```python
from build123d import *

# Parameters (mm, degrees)
SKETCH001_W = 6.3
SKETCH001_H = 1.5


with BuildPart() as y_belt_seg2:
    # Sweep001: sweep along a path in Sketch002
    with BuildLine(Plane.YZ) as sweep001_path:
        Line((-16.5, 34.3), (-2, 34.3))
        ThreePointArc((-2, 34.3), (-1.787868, 34.212132), (-1.7, 34))
        Line((-1.7, 34), (-1.7, 25.1))
        ThreePointArc((-1.7, 25.1), (-1.787868, 24.887868), (-2, 24.8))
        Line((-2, 24.8), (-16.5, 24.8))
        ThreePointArc((-16.5, 24.8), (-16.821394, 24.916978), (-16.992404, 25.213176))
        Line((-16.992404, 25.213176), (-18.285606, 32.547297))
        ThreePointArc((-18.285606, 32.547297), (-18.969647, 33.732089), (-20.255221, 34.2))
        Line((-20.255221, 34.2), (-32.255221, 34.2))
    # Sketch001 → Sweep001 (sweep)
    with BuildSketch(Plane(origin=(0, -16.5, 35.05), x_dir=(1, 0, 0), z_dir=(0, -1, 0))):
        Rectangle(SKETCH001_W, SKETCH001_H)
    sweep(path=sweep001_path.line)


with BuildPart() as part_mirroring:
    # Part__Mirroring: instance of y-belt-seg2
    add(y_belt_seg2.part.mirror(Plane(origin=(0, 0, 0), x_dir=(1, 0, 0), z_dir=(0, 1, 0))))


with BuildPart() as y_belt:
    # Sweep: sweep along a path in Sketch
    with BuildLine(Plane.YZ) as sweep_path:
        Line((16.5, 34.3), (131.990476, 34.499992))
        ThreePointArc((131.990476, 34.499992), (137.49996, 29.021053), (132.032583, 23.500097))
        Line((132.032583, 23.500097), (-138.041883, 21.900109))
        ThreePointArc((-138.041883, 21.900109), (-144.278585, 28.081635), (-138.078613, 34.3))
        Line((-138.078613, 34.3), (-16.5, 34.3))
    # Sketch001 → Sweep (sweep)
    with BuildSketch(Plane(origin=(0, -16.5, 35.05), x_dir=(1, 0, 0), z_dir=(0, -1, 0))):
        Rectangle(SKETCH001_W, SKETCH001_H)
    sweep(path=sweep_path.line)

    # Fusion: union Part__Mirroring, y-belt-seg2
    add(part_mirroring.part)
    add(y_belt_seg2.part)


solid = y_belt.part
```
Source: CAD feature listing. Evaluate the final solid. Frame: model axes, mm. A direction names the side the tool comes from. Round coordinates to 2 decimals unless told otherwise and drop trailing zeros. Write each loop counter-clockwise with the first axis right and the second up, starting at its lowest first coordinate (ties: lowest second). Pieces come first, ordered by that corner, then holes. Notation, with made-up numbers: M 32.25,-29 L 57.25,-29 A14 ccw 57.25,-21 Z; hole C 33,72.5 d10. An arc over 180 degrees is marked long. Answer as a JSON object with one key per item and string values. Group by question number.
(1) Section query B-B on y = -66.5. Output: boundary loops of the cut face in (x, z), then the cut area to 3 significant figures.
(2) Section query A-A on z = 28.1. Output: boundary loops of the cut face in (x, y).
(3) First-contact query: pin 1 (1.9 mm diameter, centred on x = 1.5, z = 31.5, fed in from +Y); pin 2 (1.9 mm diameter, centred on x = -0.5, y = 10, fed in from -Z); pin 3 (1.5 mm diameter, centred on x = 2, y = 66, fed in from +Z). Flat tips, straight axial feed; report the tip coordinate or a pass-through.
(4) Section query C-C on y = -10. Output: boundary loops of the cut face in (x, z), then the cut area to 3 significant figures.
(5) Reachability of faces 1 (the flat face through (0, -0.2, 29)), 2 (the flat face through (0, 9, 34.3)) from +Z, -Z, +X, -X, +Y, -Y: full face, straight path, thin tool, end or side. Return the list, or none.
(6) Ray query, line 1 (Z direction, x = 2, y = -132); line 2 (Z direction, x = -2.5, y = 8); line 3 (Y direction, x = 2, z = 31.5). Return the intervals inside material, ascending. Write a range as [from, to].
Computed values:
{
 "1": {"outline": "M -3.15,20.82 L 3.15,20.82 L 3.15,22.32 L -3.15,22.32 Z; M -3.15,34.3 L 3.15,34.3 L 3.15,35.8 L -3.15,35.8 Z", "area": "18.9 mm^2"},
 "2": {"outline": "M -3.15,-145.78 L 3.15,-145.78 L 3.15,-144.28 L -3.15,-144.28 Z; M -3.15,-19.02 L 3.15,-19.02 L 3.15,-17.5 L -3.15,-17.5 Z; M -3.15,-1.7 L 3.15,-1.7 L 3.15,-0.2 L -3.15,-0.2 Z; M -3.15,0.2 L 3.15,0.2 L 3.15,1.7 L -3.15,1.7 Z; M -3.15,17.5 L 3.15,17.5 L 3.15,19.02 L -3.15,19.02 Z; M -3.15,137.43 L 3.15,137.43 L 3.15,138.94 L -3.15,138.94 Z"},
 "3": {"pin 1": "y = 138.83", "pin 2": "z = 21.27", "pin 3": "z = 35.89"},
 "4": {"outline": "M -3.15,21.16 L 3.15,21.16 L 3.15,22.66 L -3.15,22.66 Z; M -3.15,23.3 L 3.15,23.3 L 3.15,24.8 L -3.15,24.8 Z; M -3.15,34.3 L 3.15,34.3 L 3.15,35.8 L -3.15,35.8 Z", "area": "28.4 mm^2"},
 "5": {"face 1": "+Z, +X, -X", "face 2": "+X, -X"},
 "6": {"line 1": "[20.44, 21.94], [34.3, 35.8]", "line 2": "[21.27, 22.77], [23.3, 24.8], [34.3, 35.8]", "line 3": "[-144.99, -143.26], [-19.62, -18.1], [-1.7, -0.2], [0.2, 1.7], [18.1, 19.62], [136.9, 138.54]"}
}
